```python
from build123d import *

# Parameters (mm, degrees)
BOSS_EXTRUDE1_DEPTH = 3
SKETCH2_W           = 15
SKETCH2_H           = 3
SKETCH2_W_2         = 3
SKETCH2_H_2         = 15
CUT_EXTRUDE1_DEPTH  = 90.073003767


with BuildPart() as part:
    # Sketch1 → Boss-Extrude1 (new body)
    with BuildSketch(Plane.XY):
        with BuildLine():
            Line((0, 0), (0, 55))
            Line((0, 55), (-40, 55))
            ThreePointArc((-40, 55), (-43.589790793, 54.333456062), (-46.701030928, 52.422680412))
            ThreePointArc((-46.701030928, 52.422680412), (-63.912940621, 28.683529165), (-70, 0))
            Line((-70, 0), (0, 0))
        make_face()
    extrude(amount=BOSS_EXTRUDE1_DEPTH)

    # Sketch2 → Cut-Extrude1 (cut, through all)
    with BuildSketch(Plane.XY.offset(3)):
        with Locations((-20, 53.5)):
            Rectangle(SKETCH2_W, SKETCH2_H)
        with Locations((-27.5, 1.5)):
            Rectangle(SKETCH2_W, SKETCH2_H)
        with Locations((-52.5, 1.5)):
            Rectangle(SKETCH2_W, SKETCH2_H)
        with Locations((-38.5, 27.5)):
            Rectangle(SKETCH2_W_2, SKETCH2_H_2)
    extrude(amount=-CUT_EXTRUDE1_DEPTH, mode=Mode.SUBTRACT)


solid = part.part
```
CAD build for the part. Positions are in the model's coordinates, mm. A direction names the side the tool comes from. Coordinates: 2 decimals unless noted, no trailing zeros. Order: outer loops, then holes, each group sorted by start corner. A loop starts at its lowest first (then second) coordinate and runs counter-clockwise, first axis right, second up. Notation, with made-up numbers: (-28, -15) - (20, -15) arc R18 ccw to (20, -2) - close; hole circle Ø6 at (1, 86). An arc over 180 degrees is marked (long way). Use a Markdown table: item, result. Add a question column.
(1) Pull direction X, two halves, no side cores. Call faces 1 (the face through (-35, 28, 3)), 2 (the face through (-53, 3, 2)), 3 (the face through (0, 27, 1)): +X half, -X half, draft (parallel to the pull), parting line (faces both ways), or undercut.
(2) Flat gauge pin, fed straight in: pin 1 (1.5 mm diameter, centred on y = 2, z = 1, fed in from -X). Where does the tip first touch, or does it go through?
(3) Saw through at C-C (x = -24). Give the cut face in (y, z).
(4) Which spindle directions (+Z, -Z, +X, -X, +Y, -Y) get a long thin tool onto all of the face, cutting with end or side? Do faces 4 (the face through (-28, 3, 2)), 5 (the face through (-20, 52, 2)), 6 (the face through (-37, 27, 2)). Say none if no direction does.
(5) Drill centre lines: line 1 along Y through (x, z) = (-38, 0.4); line 2 along Y through (x, z) = (-22.5, 0.85); line 3 along X through (y, z) = (27.5, 2). Where is each one in solid material? Low to high. Write a range as [from, to].
(6) Saw through at A-A (z = 2.5). Give the cut face in (x, y) (3 decimals), then the cut area to 3 significant figures.
(7) Saw through at B-B (y = 22). Give the cut face in (x, z).
(8) Saw through at D-D (y = 32). Give the cut face in (x, z), then the cut area to 3 significant figures.
Solved:
| question | item | result |
|---|---|---|
| 1 | face 1 | draft |
| 1 | face 2 | undercut |
| 1 | face 3 | +X half |
| 2 | pin 1 | stops at x = -69.99 |
| 3 | outline | (3, 0) - (52, 0) - (52, 3) - (3, 3) - close |
| 4 | face 4 | +Z, -Z, -Y |
| 4 | face 5 | +Z, -Z, +Y |
| 4 | face 6 | +Z, -Z |
| 5 | line 1 | y = [0, 20], [35, 55] |
| 5 | line 2 | y = [3, 52] |
| 5 | line 3 | x = [-64.43, -40], [-37, 0] |
| 6 | outline | (-70, 0) - (-60, 0) - (-60, 3) - (-45, 3) - (-45, 0) - (-35, 0) - (-35, 3) - (-20, 3) - (-20, 0) - (0, 0) - (0, 55) - (-12.5, 55) - (-12.5, 52) - (-27.5, 52) - (-27.5, 55) - (-40, 55) arc R10 ccw to (-46.701, 52.423) arc R70.625 ccw to start; hole (-40, 20) - (-37, 20) - (-37, 35) - (-40, 35) - close |
| 6 | area | 3,230 mm² |
| 7 | outline | (-66.49, 0) - (-40, 0) - (-40, 3) - (-66.49, 3) - close; (-37, 0) - (0, 0) - (0, 3) - (-37, 3) - close |
| 8 | outline | (-62.33, 0) - (-40, 0) - (-40, 3) - (-62.33, 3) - close; (-37, 0) - (0, 0) - (0, 3) - (-37, 3) - close |
| 8 | area | 178 mm² |
